Input: part model. Units: mm. Frame: model coordinates. A direction names the side the tool comes from. Round coordinates to 2 decimals unless told otherwise and drop trailing zeros. Order: outer loops, then holes, each group sorted by start corner. A loop starts at its lowest first (then second) coordinate and runs counter-clockwise, first axis right, second up. Notation, with made-up numbers: (48.5, -22.5) -> (97.5, -22.5) arc R26 cw to (97.5, 9.5) -> close; hole circle Ø10 at (-26, 4). An arc over 180 degrees is marked (long way). Answer as CSV lines item,"result". Start each with the question number.
1) Section query A-A, the plane z = 9. Output: boundary loops of the cut face in (x, y), and give its area (3 significant figures).
2) Access query for faces 4 (the face through (-4, 53.702, 18)), 5 (the face through (-22.67, -0.26, 2.46)), 6 (the face through (-6.701, 46, 3)), 7 (the face through (5.299, 46, 3)), 8 (the face through (0.799, 56, 18)). Directions: +Z, -Z, +X, -X, +Y, -Y. A direction counts if a zero-diameter tool reaches every point of the face in a straight line with its end or side. Return the directions, or none.
3) Section query B-B, the plane y = 27.5. Output: boundary loops of the cut face in (x, z), and give its area (3 significant figures).
4) Mould query, pull axis X, two halves, no side actions, for faces 1 (the face through (26.53, 7.63, 2.46)), 2 (the face through (3, 53.702, 18)), 3 (the face through (-2.201, 56, 18)). Classes: +X half, -X half, draft (parallel to the pull), parting line (faces both ways), or undercut.
5) Section query C-C, the plane x = -28. Output: boundary loops of the cut face in (y, z), and give its area (3 significant figures).
6) Line query: L1, parallel to X at y = 54, z = 18; L2, parallel to Z at x = 5, y = 23. Output: solid intervals per line, ascending.
7) First-contact query: P1, Ø2.5, axis at y = 55.5, z = 23, coming from the +X side; P2, Ø5, axis at x = 2.5, z = 24, coming from the -Y side; P3, Ø8, axis at x = 5.5, y = 10, coming from the +Z side. Flat tips, straight axial feed; report the tip coordinate or a pass-through.
```python
from build123d import *

# Parameters (mm, degrees)
F0_W     = 3
F0_H     = 5
F1_DEPTH = 5
F0_W_2   = 4.5
F2_DEPTH = 32


with BuildPart() as f1:
    # F0 (on Top) → F1 (new body)
    with BuildSketch(Plane.XY):
        with BuildLine():
            Line((47.181574, -2.732137), (5.298654, 18.285511))
            Line((5.298654, 18.285511), (5.298654, 14.702181))
            Line((5.298654, 14.702181), (0.673427, 14.702181))
            ThreePointArc((0.673427, 14.702181), (-0.701346, 14.002181), (-2.076119, 14.702181))
            Line((-2.076119, 14.702181), (-6.701346, 14.702181))
            Line((-6.701346, 14.702181), (-6.701346, 17.523266))
            Line((-6.701346, 17.523266), (-47.181575, -11.887342))
            Line((-47.181575, -11.887342), (-46.924376, -12.316116))
            Line((-46.924376, -12.316116), (-46.663222, -12.742492))
            Line((-46.663222, -12.742492), (-46.398134, -13.166434))
            Line((-46.398134, -13.166434), (-46.129137, -13.587906))
            Line((-46.129137, -13.587906), (-45.856253, -14.006872))
            Line((-45.856253, -14.006872), (-45.579504, -14.423295))
            Line((-45.579504, -14.423295), (-45.298916, -14.837141))
            Line((-45.298916, -14.837141), (-45.014511, -15.248374))
            Line((-45.014511, -15.248374), (-44.726314, -15.656958))
            Line((-44.726314, -15.656958), (-44.434351, -16.062858))
            Line((-44.434351, -16.062858), (-44.138645, -16.466041))
            Line((-44.138645, -16.466041), (-43.839222, -16.866471))
            Line((-43.839222, -16.866471), (-43.536108, -17.264114))
            Line((-43.536108, -17.264114), (-43.229328, -17.658936))
            Line((-43.229328, -17.658936), (-42.91891, -18.050904))
            Line((-42.91891, -18.050904), (-42.604879, -18.439983))
            Line((-42.604879, -18.439983), (-42.287262, -18.826141))
            Line((-42.287262, -18.826141), (-41.966087, -19.209344))
            Line((-41.966087, -19.209344), (-41.641381, -19.58956))
            Line((-41.641381, -19.58956), (-41.313171, -19.966756))
            Line((-41.313171, -19.966756), (-40.981487, -20.3409))
            Line((-40.981487, -20.3409), (-40.658041, -20.699137))
            Line((-40.658041, -20.699137), (-33.282088, -20.482399))
            Line((-33.282088, -20.482399), (-33.651937, -20.145932))
            Line((-33.651937, -20.145932), (-34.01831, -19.805685))
            Line((-34.01831, -19.805685), (-34.38117, -19.461693))
            Line((-34.38117, -19.461693), (-34.740479, -19.113994))
            Line((-34.740479, -19.113994), (-35.096199, -18.762623))
            Line((-35.096199, -18.762623), (-35.448292, -18.407618))
            Line((-35.448292, -18.407618), (-35.79672, -18.049016))
            Line((-35.79672, -18.049016), (-36.141448, -17.686856))
            Line((-36.141448, -17.686856), (-36.482439, -17.321174))
            Line((-36.482439, -17.321174), (-36.819657, -16.95201))
            Line((-36.819657, -16.95201), (-37.153067, -16.579403))
            Line((-37.153067, -16.579403), (-37.482632, -16.203392))
            Line((-37.482632, -16.203392), (-37.808319, -15.824017))
            Line((-37.808319, -15.824017), (-38.130094, -15.441317))
            Line((-38.130094, -15.441317), (-38.447921, -15.055333))
            Line((-38.447921, -15.055333), (-38.761768, -14.666106))
            Line((-38.761768, -14.666106), (-39.071602, -14.273677))
            Line((-39.071602, -14.273677), (-39.37739, -13.878087))
            Line((-39.37739, -13.878087), (-39.6791, -13.479377))
            Line((-39.6791, -13.479377), (-39.976699, -13.077591))
            Line((-39.976699, -13.077591), (-40.093318, -12.917762))
            Line((-40.093318, -12.917762), (-4.746431, 12.763255))
            Line((-4.746431, 12.763255), (-4.432819, 12.374102))
            Line((-4.432819, 12.374102), (-4.081924, 12.018203))
            Line((-4.081924, 12.018203), (-3.697251, 11.699113))
            Line((-3.697251, 11.699113), (-3.282644, 11.42002))
            Line((-3.282644, 11.42002), (-2.842246, 11.183714))
            Line((-2.842246, 11.183714), (-2.380456, 10.992554))
            Line((-2.380456, 10.992554), (-1.901889, 10.848451))
            Line((-1.901889, 10.848451), (-1.411327, 10.752845))
            Line((-1.411327, 10.752845), (-0.913671, 10.706691))
            Line((-0.913671, 10.706691), (-0.413894, 10.710451))
            Line((-0.413894, 10.710451), (0.083012, 10.764086))
            Line((0.083012, 10.764086), (0.57208, 10.867061))
            Line((0.57208, 10.867061), (1.048425, 11.018347))
            Line((1.048425, 11.018347), (1.507287, 11.216432))
            Line((1.507287, 11.216432), (1.94408, 11.459338))
            Line((1.94408, 11.459338), (2.354442, 11.744636))
            Line((2.354442, 11.744636), (2.734271, 12.069477))
            Line((2.734271, 12.069477), (3.079772, 12.430615))
            Line((3.079772, 12.430615), (3.387494, 12.824441))
            Line((3.387494, 12.824441), (3.654361, 13.247021))
            Line((3.654361, 13.247021), (3.767534, 13.459612))
            Line((3.767534, 13.459612), (40.612321, -5.029804))
            Line((40.612321, -5.029804), (40.385651, -5.47547))
            Line((40.385651, -5.47547), (40.154175, -5.918659))
            Line((40.154175, -5.918659), (39.917917, -6.359317))
            Line((39.917917, -6.359317), (39.676907, -6.797395))
            Line((39.676907, -6.797395), (39.431173, -7.23284))
            Line((39.431173, -7.23284), (39.180743, -7.665601))
            Line((39.180743, -7.665601), (38.925647, -8.095628))
            Line((38.925647, -8.095628), (38.665914, -8.522871))
            Line((38.665914, -8.522871), (38.401574, -8.947279))
            Line((38.401574, -8.947279), (38.13266, -9.368803))
            Line((38.13266, -9.368803), (37.859202, -9.787394))
            Line((37.859202, -9.787394), (37.581232, -10.203002))
            Line((37.581232, -10.203002), (37.298782, -10.615579))
            Line((37.298782, -10.615579), (37.011887, -11.025077))
            Line((37.011887, -11.025077), (36.720579, -11.431448))
            Line((36.720579, -11.431448), (36.424892, -11.834644))
            Line((36.424892, -11.834644), (36.124861, -12.234618))
            Line((36.124861, -12.234618), (35.820522, -12.631323))
            Line((35.820522, -12.631323), (35.511909, -13.024713))
            Line((35.511909, -13.024713), (35.399096, -13.166355))
            Line((35.399096, -13.166355), (35.567373, -20.590768))
            Line((35.567373, -20.590768), (35.919316, -20.235615))
            Line((35.919316, -20.235615), (36.267782, -19.87705))
            Line((36.267782, -19.87705), (36.612738, -19.515105))
            Line((36.612738, -19.515105), (36.95415, -19.149817))
            Line((36.95415, -19.149817), (37.291986, -18.781218))
            Line((37.291986, -18.781218), (37.626214, -18.409345))
            Line((37.626214, -18.409345), (37.956803, -18.034233))
            Line((37.956803, -18.034233), (38.28372, -17.655917))
            Line((38.28372, -17.655917), (38.606936, -17.274433))
            Line((38.606936, -17.274433), (38.926418, -16.889818))
            Line((38.926418, -16.889818), (39.242138, -16.502108))
            Line((39.242138, -16.502108), (39.554064, -16.111339))
            Line((39.554064, -16.111339), (39.862168, -15.71755))
            Line((39.862168, -15.71755), (40.166419, -15.320776))
            Line((40.166419, -15.320776), (40.46679, -14.921057))
            Line((40.46679, -14.921057), (40.763251, -14.51843))
            Line((40.763251, -14.51843), (41.055775, -14.112933))
            Line((41.055775, -14.112933), (41.344333, -13.704604))
            Line((41.344333, -13.704604), (41.628898, -13.293483))
            Line((41.628898, -13.293483), (41.909444, -12.879608))
            Line((41.909444, -12.879608), (42.185943, -12.46302))
            Line((42.185943, -12.46302), (42.45837, -12.043756))
            Line((42.45837, -12.043756), (42.726698, -11.621858))
            Line((42.726698, -11.621858), (42.990902, -11.197365))
            Line((42.990902, -11.197365), (43.250957, -10.770318))
            Line((43.250957, -10.770318), (43.506838, -10.340757))
            Line((43.506838, -10.340757), (43.758521, -9.908722))
            Line((43.758521, -9.908722), (44.005982, -9.474256))
            Line((44.005982, -9.474256), (44.249197, -9.037398))
            Line((44.249197, -9.037398), (44.488144, -8.598192))
            Line((44.488144, -8.598192), (44.722799, -8.156678))
            Line((44.722799, -8.156678), (44.953141, -7.712898))
            Line((44.953141, -7.712898), (45.179148, -7.266894))
            Line((45.179148, -7.266894), (45.400797, -6.818709))
            Line((45.400797, -6.818709), (45.618069, -6.368386))
            Line((45.618069, -6.368386), (45.830942, -5.915967))
            Line((45.830942, -5.915967), (46.039396, -5.461495))
            Line((46.039396, -5.461495), (46.243411, -5.005013))
            Line((46.243411, -5.005013), (46.442969, -4.546565))
            Line((46.442969, -4.546565), (46.638049, -4.086193))
            Line((46.638049, -4.086193), (46.828634, -3.623943))
            Line((46.828634, -3.623943), (47.014706, -3.159858))
            Line((47.014706, -3.159858), (47.181574, -2.732137))
        make_face()
        with BuildLine():
            Line((5.298654, 14.702181), (5.298654, 18.285511))
            Line((5.298654, 18.285511), (1.541223, 20.171061))
            Line((1.541223, 20.171061), (1.083876, 20.372618))
            Line((1.083876, 20.372618), (0.608691, 20.52751))
            Line((0.608691, 20.52751), (0.120418, 20.634189))
            Line((0.120418, 20.634189), (-0.376067, 20.691589))
            Line((-0.376067, 20.691589), (-0.875802, 20.699137))
            Line((-0.875802, 20.699137), (-1.373793, 20.656756))
            Line((-1.373793, 20.656756), (-1.865066, 20.564871))
            Line((-1.865066, 20.564871), (-2.344711, 20.4244))
            Line((-2.344711, 20.4244), (-2.807936, 20.236746))
            Line((-2.807936, 20.236746), (-3.250113, 20.003784))
            Line((-3.250113, 20.003784), (-3.640272, 19.747266))
            Line((-3.640272, 19.747266), (-6.701346, 17.523266))
            Line((-6.701346, 17.523266), (-6.701346, 14.702181))
            Line((-6.701346, 14.702181), (-2.076119, 14.702181))
            ThreePointArc((-2.076119, 14.702181), (-1.227125, 17.318831), (0.998654, 15.702181))
            ThreePointArc((0.998654, 15.702181), (0.915304, 15.176402), (0.673427, 14.702181))
            Line((0.673427, 14.702181), (5.298654, 14.702181))
        make_face()
        Polygon((5.298654, 53.702181), (0.798654, 53.702181), (-2.201346, 53.702181), (-6.701346, 53.702181), (-6.701346, 17.523266), (-3.640272, 19.747266), (-3.250113, 20.003784), (-2.807936, 20.236746), (-2.344711, 20.4244), (-1.865066, 20.564871), (-1.373793, 20.656756), (-0.875802, 20.699137), (-0.376067, 20.691589), (0.120418, 20.634189), (0.608691, 20.52751), (1.083876, 20.372618), (1.541223, 20.171061), (5.298654, 18.285511), align=None)
        with Locations((-0.701346, 56.202181)):
            Rectangle(F0_W, F0_H)
    extrude(amount=F1_DEPTH)

    # F0 (on Top) → F2 (join)
    with BuildSketch(Plane.XY):
        with Locations((-4.451346, 56.202181)):
            Rectangle(F0_W_2, F0_H)
        with Locations((3.048654, 56.202181)):
            Rectangle(F0_W_2, F0_H)
    extrude(amount=F2_DEPTH)


solid = f1.part
```
Findings:
1,outline,"(-6.7, 53.7) -> (-2.2, 53.7) -> (-2.2, 58.7) -> (-6.7, 58.7) -> close; (0.8, 53.7) -> (5.3, 53.7) -> (5.3, 58.7) -> (0.8, 58.7) -> close"
1,area,"45.0 mm^2"
2,face 4,"+Z, +X, -X, -Y"
2,face 5,"+Z, -Z"
2,face 6,"+Z, -Z, -X, +Y"
2,face 7,"+Z, -Z, +X, +Y"
2,face 8,"+Z, +Y, -Y"
3,outline,"(-6.7, 0) -> (5.3, 0) -> (5.3, 5) -> (-6.7, 5) -> close"
3,area,"60.0 mm^2"
4,face 1,"+X half"
4,face 2,"draft"
4,face 3,"undercut"
5,outline,"(-4.13, 0) -> (2.05, 0) -> (2.05, 5) -> (-4.13, 5) -> close"
5,area,"30.9 mm^2"
6,L1,"x = -6.7 to -2.2, 0.8 to 5.3"
6,L2,"z = 0 to 5"
7,P1,"stops at x = 5.3"
7,P2,"stops at y = 53.7"
7,P3,"stops at z = 5"
